Input: dimensioned drawing with shaded views. Units: mm. Origin: part minimum x, y, z. A direction names the side the tool comes from. Give positions to 0.01 mm unless a question says otherwise; leave off trailing zeros. Order: outer loops, then holes, each group sorted by start corner. A loop starts at its lowest first (then second) coordinate and runs counter-clockwise, first axis right, second up. Notation, with made-up numbers: (-10.75, 55) -> (47.25, 55) arc R26 cw to (47.25, 91) -> close; hole circle Ø8 at (-21.75, 31.25). An arc over 180 degrees is marked (long way). Use CSV: the item, a comma, the result in double quotes.
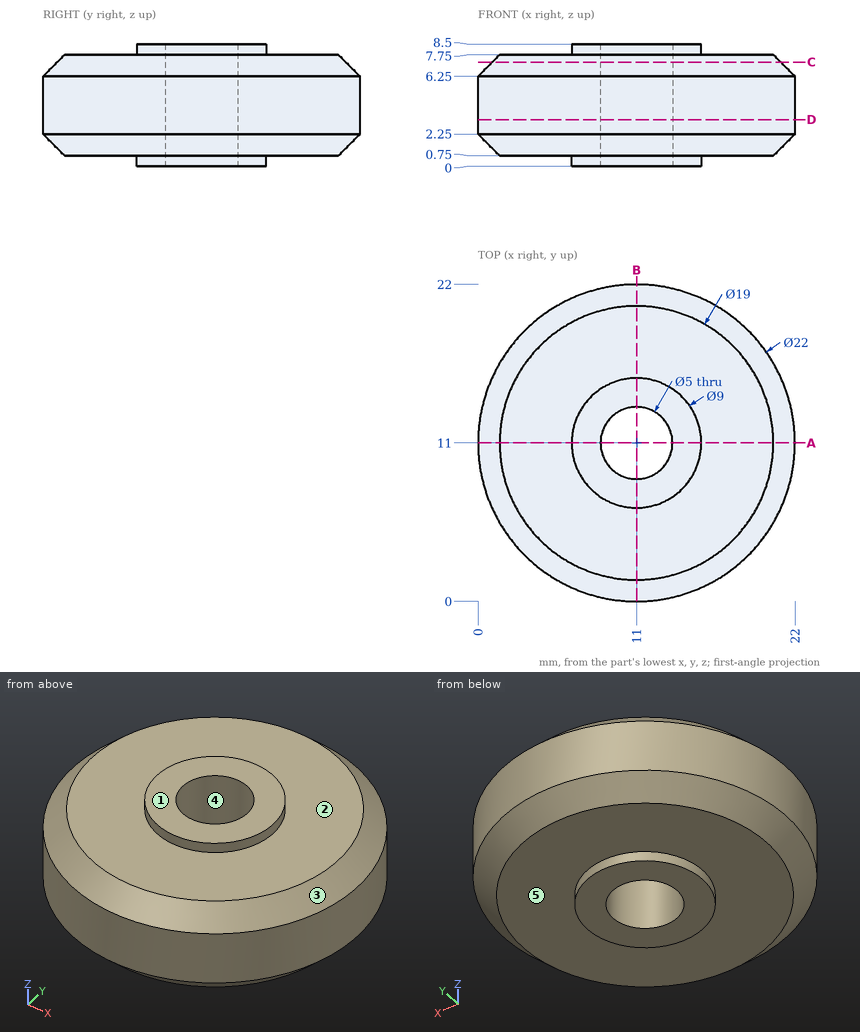
1. Section query D-D on z = 3.25. Return loops of the section in (x, y).
Answer below:
outline,"circle Ø22 at (11, 11); hole circle Ø5 at (11, 11)"
2. Ray query, line 1 along Y through (x, z) = (11, 5.5); line 2 along Z through (x, y) = (3.5, 16.25); line 3 along Y through (x, z) = (11, 2). Return the intervals inside material, ascending.
Answer below:
line 1,"y = 0 to 8.5, 13.5 to 22"
line 2,"z = 0.75 to 7.75"
line 3,"y = 0.25 to 8.5, 13.5 to 21.75"
3. Mould query, pull axis Y, two halves, no side actions, for the marked faces 3, 4 and 5. Classes: released by +Y, released by -Y, zero draft, split by the parting line, or undercut.
Answer below:
face 3,"split by the parting line"
face 4,"undercut"
face 5,"zero draft"
4. Pin query (flat end, axial travel): P1, Ø9.5, axis at x = 15, y = 7, coming from the +Z side; P2, Ø3, axis at x = 7.5, z = 4, coming from the +Y side; P3, Ø4, axis at x = 4.5, y = 8.5, coming from the +Z side; P4, Ø2, axis at x = 7.5, z = 2.5, coming from the +Y side. Return the tip coordinate at first contact, or that it passes through.
Answer below:
P1,"stops at z = 8.5"
P2,"stops at y = 21.82"
P3,"stops at z = 7.75"
P4,"stops at y = 21.71"
5. Section query A-A on y = 11. Return loops of the section in (x, z).
Answer below:
outline,"(0, 2.25) -> (1.5, 0.75) -> (6.5, 0.75) -> (6.5, 0) -> (8.5, 0) -> (8.5, 8.5) -> (6.5, 8.5) -> (6.5, 7.75) -> (1.5, 7.75) -> (0, 6.25) -> close; (13.5, 0) -> (15.5, 0) -> (15.5, 0.75) -> (20.5, 0.75) -> (22, 2.25) -> (22, 6.25) -> (20.5, 7.75) -> (15.5, 7.75) -> (15.5, 8.5) -> (13.5, 8.5) -> close"
6. Access query for the marked faces 1 and 2. Directions: +Z, -Z, +X, -X, +Y, -Y. A direction counts if a zero-diameter tool reaches every point of the face in a straight line with its end or side. Return the directions, or none.
Answer below:
face 1,"+Z, +X, -X, +Y, -Y"
face 2,"+Z"
7. Section query C-C on z = 7.25. Return loops of the section in (x, y).
Answer below:
outline,"circle Ø20 at (11, 11); hole circle Ø5 at (11, 11)"
